Model file for the job. Use its own axes, mm. A direction names the side the tool comes from. Coordinates: 2 decimals unless noted, no trailing zeros. Write each loop counter-clockwise with the first axis right and the second up, starting at its lowest first coordinate (ties: lowest second). Pieces come first, ordered by that corner, then holes. Notation, with made-up numbers: (44, 75) -> (86, 75) arc R13 ccw to (86, 82) -> close; hole circle Ø9 at (-28.5, 52.5). An arc over 180 degrees is marked (long way). Answer as a JSON object with one key per item and string values. Group by question number.
from build123d import *

# Parameters (mm, degrees)
F0_W     = 57.15
F0_H     = 203.2
F1_DEPTH = 88.9
F0_H_2   = 57.15
F0_R     = 19.685
F2_DEPTH = 6.35
F3_W     = 6.35
F3_H     = 57.15
F4_DEPTH = 57.15
F5_R     = 19.685
F6_DEPTH = 6.35
F7_SIZE2 = 165.8896583964
F7_SIZE  = 44.45


with BuildPart() as f1:
    # F0 (on Right) → F1 (new body)
    with BuildSketch(Plane.YZ):
        with Locations((0, -130.175)):
            Rectangle(F0_W, F0_H)
    extrude(amount=F1_DEPTH)

    # F0 (on Right) → F2 (join)
    with BuildSketch(Plane.YZ):
        Rectangle(F0_W, F0_H_2)
        Circle(F0_R, mode=Mode.SUBTRACT)
    extrude(amount=F2_DEPTH)

    # F3 (on face) → F4 (join)
    with BuildSketch(Plane.XY.offset(-28.575)):
        with Locations((85.725, 0)):
            Rectangle(F3_W, F3_H)
    extrude(amount=F4_DEPTH)

    # F5 (on face) → F6 (cut)
    with BuildSketch(Plane(origin=(82.55, 0, 0), x_dir=(0, -1, 0), z_dir=(-1, 0, 0))):
        Circle(F5_R)
    extrude(amount=-F6_DEPTH, mode=Mode.SUBTRACT)

    # F7
    f7_edges = [f1.edges().sort_by_distance(p)[0] for p in [
        (44.45, -28.575, -231.775),
    ]]
    f7_side = f1.faces().sort_by_distance((44.45, 0, -231.775))[0]
    chamfer(f7_edges, length=F7_SIZE, length2=F7_SIZE2, reference=f7_side)


solid = f1.part
(1) Cut at B-B on y = 6. List the corners of the cut face in (x, z) (3 decimals).
(2) 3-axis set-ups, long thin cutter, end or side, ignore diameter. For faces 1 (the face through (6.35, -7, 19)), 2 (the face through (86, 0, 28.575)): which of +Z, -Z, +X, -X, +Y, -Y reach the whole face in a straight line?
(3) Cut at A-A on z = 0. List the corners of the cut face in (x, y) (3 decimals).
(4) Cut at D-D on x = 52.5. List the corners of the cut face in (y, z) (3 decimals).
(5) Wall check: probe 1 along X at (y, z) = (7, -27); probe 2 along Z at (x, y) = (26, 16) (3 decimals); probe 3 along Y at (x, z) = (30.5, -76) (3 decimals). Give the ranges that are in metal, low to high.
(6) Pin check, flat tip, straight feed: pin 1 (2 mm diameter, centred on x = 31.5, y = 6.5, fed in from +Z) (3 decimals). Stop position of the tip, or through.
(7) Pull direction Y, two halves, no side cores. Call faces 3 (the face through (44, 28.575, -132)), 4 (the face through (3.13, -15.62, -11.98)), 5 (the face through (85.68, 15.62, -11.98)), 6 (the face through (44, -28.575, -40)): released by +Y, released by -Y, zero draft, split by the parting line, or undercut.
(8) Cut at C-C on y = 22.5. List the corners of the cut face in (x, z) (3 decimals).
Results found:
{
 "1": {"outline": "(0, -194.921) -> (88.9, -194.921) -> (88.9, -18.748) -> (82.55, -18.748) -> (82.55, -28.575) -> (6.35, -28.575) -> (6.35, -18.748) -> (0, -18.748) -> close; (0, 18.748) -> (6.35, 18.748) -> (6.35, 28.575) -> (0, 28.575) -> close; (82.55, 18.748) -> (88.9, 18.748) -> (88.9, 28.575) -> (82.55, 28.575) -> close"},
 "2": {"face 1": "+Z, +Y, -Y", "face 2": "+Z, +X, -X, +Y, -Y"},
 "3": {"outline": "(0, -28.575) -> (6.35, -28.575) -> (6.35, -19.685) -> (0, -19.685) -> close; (0, 19.685) -> (6.35, 19.685) -> (6.35, 28.575) -> (0, 28.575) -> close; (82.55, -28.575) -> (88.9, -28.575) -> (88.9, -19.685) -> (82.55, -19.685) -> close; (82.55, 19.685) -> (88.9, 19.685) -> (88.9, 28.575) -> (82.55, 28.575) -> close"},
 "4": {"outline": "(-28.575, -65.885) -> (15.875, -231.775) -> (28.575, -231.775) -> (28.575, -28.575) -> (-28.575, -28.575) -> close"},
 "5": {"probe 1": "x = 0 to 6.35, 82.55 to 88.9", "probe 2": "z = -231.775 to -28.575", "probe 3": "y = -25.865 to 28.575"},
 "6": {"pin 1": "stops at z = -28.575"},
 "7": {"face 3": "released by +Y", "face 4": "undercut", "face 5": "undercut", "face 6": "released by -Y"},
 "8": {"outline": "(0, -231.775) -> (88.9, -231.775) -> (88.9, 28.575) -> (82.55, 28.575) -> (82.55, -28.575) -> (6.35, -28.575) -> (6.35, 28.575) -> (0, 28.575) -> close"}
}
